Autodesk Inventor part; units mm, degrees
ref_plane "YZ Plane" through (0, 0, 0) normal (1, 0, 0) x (0, 1, 0)
ref_plane "XZ Plane" through (0, 0, 0) normal (0, 1, 0) x (-1, 0, 0)
ref_plane "XY Plane" through (0, 0, 0) normal (0, 0, 1) x (1, 0, 0)
sketch "Sketch1" plane through (0, 0, 0) normal (0, 1, 0) x (-1, 0, 0)
  line L0 (23.5265, 54.5795) -> (-113.4735, 54.5795)
  line L1 (-113.4735, 54.5795) -> (-113.4735, -435.4205)
  line L2 (-113.4735, -435.4205) -> (23.5265, -435.4205)
  line L3 (23.5265, -435.4205) -> (23.5265, 54.5795)
  point P0 (0, 0)
  dimension "d0" = 137
  dimension "d1" = 490
extrude "Extrusion1" add sketch "Sketch1" along normal blind 15
sketch "Sketch2" plane through (-23.5265, 0, 54.5795) normal (0, 0, 1) x (1, 0, 0)
  line L0 (137, 0) -> (0, 0)
  line L1 (0, 0) -> (127, 0)
  line L2 (127, 0) -> (127, 5)
  line L3 (127, 5) -> (0, 5)
  line L4 (0, 5) -> (0, 0)
  point P0 (23.5265, 0)
  dimension "d4" = 127
  dimension "d5" = 5
extrude "Extrusion2" cut sketch "Sketch2" against normal blind 7
sketch "Sketch3" plane through (113.4735, 0, -435.4205) normal (0, 0, -1) x (-1, 0, 0)
  line L0 (0, 0) -> (137, 0)
  line L1 (0, 0) -> (137, 0)
  line L2 (137, 0) -> (137, 5)
  line L3 (137, 5) -> (0, 5)
  line L4 (0, 5) -> (0, 0)
  point P0 (113.4735, 0)
  dimension "d8" = 137
  dimension "d9" = 5
extrude "Extrusion3" cut sketch "Sketch3" against normal blind 7
sketch "Sketch4" plane through (0, 0, 0) normal (0, -1, 0) x (1, 0, 0)
  line L0 (-23.5265, -428.4205) -> (113.4735, -428.4205)
  line L1 (103.4735, 47.5795) -> (-23.5265, 47.5795)
  line L2 (113.4735, -428.4205) -> (103.4735, -428.4205)
  line L3 (103.4735, -428.4205) -> (103.4735, 47.5795)
  line L4 (103.4735, 47.5795) -> (113.4735, 47.5795)
  line L5 (113.4735, 47.5795) -> (113.4735, -428.4205)
  point P0 (0, 0)
  point P1 (-13.5265, -428.4205)
  dimension "d12" = 10
  dimension "d13" = 476
extrude "Extrusion4" cut sketch "Sketch4" against normal blind 5
sketch "Sketch5" plane through (0, 15, 0) normal (0, 1, 0) x (1, 0, 0)
  circle A0 centre (22.1402, 68.4205) radius 15
  circle A1 centre (67.8068, 128.4205) radius 15
  circle A2 centre (44.9735, 228.4205) radius 20
  line L0 (103.4735, 428.4205) -> (-23.5265, 428.4205)
  line L1 (-23.5265, 435.4205) -> (-23.5265, -54.5795)
  point P0 (0, 0)
  point P1 (-13.5265, 428.4205)
  dimension "d16" = 40
  dimension "d17" = 200
  dimension "d18" = 68.5
  dimension "d19" = 300
  dimension "d20" = 91.3333
  dimension "d21" = 45.6667
  dimension "d22" = 360
  dimension "d23" = 30
  dimension "d24" = 30
extrude "Extrusion5" cut sketch "Sketch5" against normal blind 15
sketch "Sketch6" plane through (0, 0, 0) normal (0, -1, 0) x (1, 0, 0)
  line L0 (69.9735, -253.4205) -> (19.9735, -253.4205)
  line L1 (19.9735, -253.4205) -> (19.9735, -203.4205)
  line L2 (19.9735, -203.4205) -> (69.9735, -203.4205)
  line L3 (69.9735, -203.4205) -> (69.9735, -253.4205)
  circle A0 centre (44.9735, -228.4205) radius 20
  point P0 (0, 0)
  dimension "d27" = 25
  dimension "d28" = 50
  dimension "d29" = 25
  dimension "d30" = 50
extrude "Extrusion6" cut sketch "Sketch6" against normal blind 12
sketch "Sketch7" plane through (0, 15, 0) normal (0, 1, 0) x (1, 0, 0)
  circle A0 centre (44.9735, 228.4205) radius 20
  point P0 (0, 0)
  point P1 (28.7235, 212.1705)
  point P2 (28.7235, 244.6705)
  point P3 (61.2235, 244.6705)
  point P4 (61.2235, 212.1705)
  dimension "d33" = 16.25
  dimension "d34" = 16.25
  dimension "d35" = 16.25
  dimension "d36" = 16.25
  dimension "d37" = 16.25
  dimension "d38" = 16.25
  dimension "d39" = 16.25
  dimension "d40" = 16.25
hole "Hole1" at (28.7235, 15, -212.1705) at (28.7235, 15, -244.6705) at (61.2235, 15, -244.6705) at (61.2235, 15, -212.1705) direction (0, -1, 0) diameter 2.5 end through all
sketch "Sketch8" plane through (0, 0, 0) normal (0, -1, 0) x (1, 0, 0)
  circle A0 centre (61.2235, -244.6705) radius 1.25
  circle A1 centre (28.7235, -212.1705) radius 1.25
  circle A2 centre (28.7235, -244.6705) radius 1.25
  circle A3 centre (61.2235, -212.1705) radius 1.25
  line L0 (19.9735, -203.4205) -> (69.9735, -203.4205)
  line L1 (19.9735, -253.4205) -> (19.9735, -203.4205)
  line L2 (69.9735, -253.4205) -> (19.9735, -253.4205)
  line L3 (69.9735, -203.4205) -> (69.9735, -253.4205)
  circle A4 centre (44.9735, -228.4205) radius 20
  line L4 (69.9735, -203.4205) -> (69.9735, -253.4205)
  line L5 (69.9735, -253.4205) -> (79.9735, -253.4205)
  line L6 (79.9735, -253.4205) -> (79.9735, -203.4205)
  line L7 (79.9735, -203.4205) -> (69.9735, -203.4205)
  line L8 (69.9735, -203.4205) -> (69.9735, -253.4205)
  line L9 (79.9735, -203.4205) -> (19.9735, -203.4205)
  line L10 (19.9735, -203.4205) -> (19.9735, -193.4205)
  line L11 (19.9735, -193.4205) -> (79.9735, -193.4205)
  line L12 (79.9735, -193.4205) -> (79.9735, -203.4205)
  point P0 (0, 0)
  dimension "d48" = 10
  dimension "d49" = 50
  dimension "d50" = 60
  dimension "d51" = 10
extrude "Extrusion7" cut sketch "Sketch8" against normal blind 12 contours L10 L11 L12 L7 L0 | L7 L6 L5 L3
sketch "Sketch9" plane through (0, 15, 0) normal (0, 1, 0) x (1, 0, 0)
  line L0 (43.4735, 338.4205) -> (83.4735, 338.4205)
  line L1 (83.4735, 338.4205) -> (83.4735, 398.4205)
  line L2 (83.4735, 398.4205) -> (43.4735, 398.4205)
  line L3 (43.4735, 398.4205) -> (43.4735, 338.4205)
  line L4 (103.4735, 428.4205) -> (-23.5265, 428.4205)
  line L5 (113.4735, -54.5795) -> (113.4735, 435.4205)
  line L6 (46.6735, 342.9072) -> (52.6735, 342.9072)
  line L7 (52.6735, 342.9072) -> (52.6735, 392.9072)
  line L8 (52.6735, 392.9072) -> (46.6735, 392.9072)
  line L9 (46.6735, 392.9072) -> (46.6735, 342.9072)
  line L10 (55.8735, 342.9072) -> (61.8735, 342.9072)
  line L11 (61.8735, 342.9072) -> (61.8735, 392.9072)
  line L12 (61.8735, 392.9072) -> (55.8735, 392.9072)
  line L13 (55.8735, 392.9072) -> (55.8735, 342.9072)
  line L14 (65.0735, 342.9072) -> (71.0735, 342.9072)
  line L15 (71.0735, 342.9072) -> (71.0735, 392.9072)
  line L16 (71.0735, 392.9072) -> (65.0735, 392.9072)
  line L17 (65.0735, 392.9072) -> (65.0735, 342.9072)
  line L18 (74.2735, 342.9072) -> (80.2735, 342.9072)
  line L19 (80.2735, 342.9072) -> (80.2735, 392.9072)
  line L20 (80.2735, 392.9072) -> (74.2735, 392.9072)
  line L21 (74.2735, 392.9072) -> (74.2735, 342.9072)
  point P0 (0, 0)
  point P1 (-13.5265, 428.4205)
  dimension "d54" = 60
  dimension "d55" = 40
  dimension "d56" = 30
  dimension "d57" = 30
  dimension "d58" = 50
  dimension "d59" = 50
  dimension "d60" = 6
  dimension "d61" = 6
  dimension "d62" = 6
  dimension "d63" = 6
  dimension "d64" = 3.2
  dimension "d65" = 3.2
  dimension "d66" = 3.2
  dimension "d67" = 3.2
extrude "Extrusion8" cut sketch "Sketch9" against normal blind 15 contours L9 L8 L7 L6 | L13 L12 L11 L10 | L17 L16 L15 L14 | L21 L20 L19 L18
sketch "Sketch11" plane through (0, 0, 0) normal (0, -1, 0) x (1, 0, 0)
  line L0 (103.4735, -400.4205) -> (23.4735, -400.4205)
  line L1 (23.4735, -400.4205) -> (23.4735, -285.4205)
  line L2 (23.4735, -285.4205) -> (103.4735, -285.4205)
  line L3 (103.4735, -285.4205) -> (103.4735, -400.4205)
  line L4 (113.4735, 47.5795) -> (113.4735, -435.4205)
  line L5 (113.4735, -435.4205) -> (-23.5265, -435.4205)
  point P0 (0, 0)
  point P1 (-13.5265, -435.4205)
  dimension "d70" = 80
  dimension "d71" = 115
  dimension "d72" = 10
  dimension "d73" = 35
extrude "Extrusion9" cut sketch "Sketch11" against normal blind 10
sketch "Sketch12" plane through (-23.5265, 15, 54.5795) normal (0, 0, 1) x (1, 0, 0)
  line L0 (0, 0) -> (137, 0)
  line L1 (137, -121) -> (137, 0)
  line L2 (127, -15) -> (137, -15)
  line L3 (127, -10) -> (127, -121)
  line L4 (0, -10) -> (127, -10)
  line L5 (127, -10) -> (127, -121)
  line L6 (0, -10) -> (127, -10)
  line L7 (137, -15) -> (137, -10)
  line L8 (127, -10) -> (137, -10)
  line L9 (137, -10) -> (137, -15)
  line L10 (137, -15) -> (127, -15)
  line L11 (127, -15) -> (127, -10)
  point P0 (23.5265, -15)
extrude "Extrusion10" cut sketch "Sketch12" against normal blind 7
sketch "Sketch13" plane through (0, 0, 0) normal (0, -1, 0) x (1, 0, 0)
  line L0 (23.4735, -285.4205) -> (103.4735, -285.4205)
  line L1 (103.4735, -285.4205) -> (103.4735, 47.5795)
  line L2 (103.4735, 47.5795) -> (-23.5265, 47.5795)
  line L3 (-23.5265, -428.4205) -> (-23.5265, 47.5795)
  line L4 (-23.5265, -428.4205) -> (103.4735, -428.4205)
  line L5 (103.4735, -428.4205) -> (103.4735, -400.4205)
  line L6 (103.4735, -400.4205) -> (23.4735, -400.4205)
  line L7 (23.4735, -400.4205) -> (23.4735, -285.4205)
  circle A0 centre (67.8068, -128.4205) radius 15
  circle A1 centre (22.1402, -68.4205) radius 15
  line L8 (19.9735, -253.4205) -> (19.9735, -193.4205)
  line L9 (19.9735, -193.4205) -> (79.9735, -193.4205)
  line L10 (79.9735, -193.4205) -> (79.9735, -253.4205)
  line L11 (79.9735, -253.4205) -> (19.9735, -253.4205)
  line L12 (-23.5265, -435.4205) -> (-23.5265, -428.4205)
  line L13 (103.4735, -285.4205) -> (103.4735, 47.5795)
  line L14 (-23.5265, -428.4205) -> (103.4735, -428.4205)
  line L15 (103.4735, -428.4205) -> (103.4735, 47.5795)
  line L16 (103.4735, 47.5795) -> (-23.5265, 47.5795)
  line L17 (-23.5265, 47.5795) -> (-23.5265, -428.4205)
  point P0 (0, 0)
extrude "Extrusion11" add sketch "Sketch13" along normal blind 1 contours L7 L6 L5 L4 L3 L2 L1 L0
properties part number "Arcade_ControlTop"
Work out the finished part from the listing and answer in its coordinate system (mm). A direction names the side the tool comes from. Round coordinates to 2 decimals unless told otherwise and drop trailing zeros. Write each loop counter-clockwise with the first axis right and the second up, starting at its lowest first coordinate (ties: lowest second). Pieces come first, ordered by that corner, then holes.
1) Determine the mould class of faces 1 (the face through (44, 10, 54.58)), 2 (the face through (18.888, 7.112, -53.777)), 3 (the face through (-23.526, 7, -194)), 4 (the face through (46, 10, -435.42)) for opening direction Z: pulls with the +Z half, pulls with the -Z half, needs draft (parallel to the pull), parting line crosses it, or undercut.
2) Consider probe 1 along Z at (x, y) = (52, 2.5); probe 2 along Z at (x, y) = (78.5, 1); probe 3 along Z at (x, y) = (30, 8.5). Determine where each line is inside the solid, lowest interval first.
3) A cutting plane is placed at B-B on x = 88. Determine the outline of the cut face in (y, z).
4) Flat-ended cylindrical pins translate along their axes: P1, Ø1.8, axis at y = 2.5, z = -413.5, coming from the +X side; P2, Ø4, axis at x = 61.5, y = 1, coming from the +Z side; P3, Ø18, axis at x = 59, z = -209.5, coming from the -Y side. Find the tip coordinate at first contact, or state that the pin passes through.
5) Which of the six approach directions +Z, -Z, +X, -X, +Y, -Y give full straight-line access (tool end or side, diameter ignored) to faces 5 (the face through (50, 6, -193.42)), 6 (the face through (40.638, 13.521, -208.896))?
6) A cutting plane is placed at A-A on z = -355. Determine the outline of the cut face in (x, y).
7) A cutting plane is placed at C-C on z = -48. Determine the outline of the cut face in (x, y).
Entries:
1. face 1: pulls with the +Z half
1. face 2: undercut
1. face 3: needs draft
1. face 4: pulls with the -Z half
2. probe 1: z = -428.42 to -400.42, -285.42 to -253.42, -193.42 to 47.58
2. probe 2: z = -428.42 to -400.42, -285.42 to -253.42, -193.42 to -138.94, -117.9 to 47.58
2. probe 3: z = -435.42 to -400.42, -285.42 to -253.42, -193.42 to -81.2, -55.64 to 54.58
3. outline: (-1, -428.42) - (5, -428.42) - (5, -435.42) - (15, -435.42) - (15, 54.58) - (5, 54.58) - (5, 47.58) - (-1, 47.58) - (-1, -285.42) - (10, -285.42) - (10, -400.42) - (-1, -400.42) - close
4. P1: stops at x = 103.47
4. P2: stops at z = 47.58
4. P3: stops at y = 12
5. face 5: -Y
5. face 6: +Y, -Y
6. outline: (-23.53, -1) - (23.47, -1) - (23.47, 10) - (46.67, 10) - (46.67, 15) - (-23.53, 15) - close; (52.67, 10) - (55.87, 10) - (55.87, 15) - (52.67, 15) - close; (61.87, 10) - (65.07, 10) - (65.07, 15) - (61.87, 15) - close; (71.07, 10) - (74.27, 10) - (74.27, 15) - (71.07, 15) - close; (80.27, 10) - (103.47, 10) - (103.47, 5) - (113.47, 5) - (113.47, 15) - (80.27, 15) - close
7. outline: (-23.53, -1) - (103.47, -1) - (103.47, 5) - (113.47, 5) - (113.47, 15) - (-23.53, 15) - close
